```python
from build123d import *

# Parameters (mm, degrees)
SKETCH1_W           = 46
SKETCH1_H           = 42
BOSS_EXTRUDE1_DEPTH = 3
SKETCH2_W           = 13
SKETCH2_H           = 3
CUT_EXTRUDE1_DEPTH  = 32.288975694
SKETCH3_W           = 3
SKETCH3_H           = 10
CUT_EXTRUDE2_DEPTH  = 32.288975694


with BuildPart() as part:
    # Sketch1 → Boss-Extrude1 (new body)
    with BuildSketch(Plane.XY):
        Rectangle(SKETCH1_W, SKETCH1_H)
    extrude(amount=BOSS_EXTRUDE1_DEPTH)

    # Sketch2 → Cut-Extrude1 (cut, through all)
    with BuildSketch(Plane.XY.offset(3)):
        with Locations((-16.5, -19.5)):
            Rectangle(SKETCH2_W, SKETCH2_H)
        with Locations((16.5, -19.5)):
            Rectangle(SKETCH2_W, SKETCH2_H)
    extrude(amount=-CUT_EXTRUDE1_DEPTH, mode=Mode.SUBTRACT)

    # Sketch3 → Cut-Extrude2 (cut, through all)
    with BuildSketch(Plane(origin=(0, 0, 0), x_dir=(-1, 0, 0), z_dir=(0, 0, -1))):
        with Locations((-21.5, 0.5)):
            Rectangle(SKETCH3_W, SKETCH3_H)
        with Locations((21.5, 0.5)):
            Rectangle(SKETCH3_W, SKETCH3_H)
    extrude(amount=-CUT_EXTRUDE2_DEPTH, mode=Mode.SUBTRACT)


solid = part.part
```
Read the model definition and answer for the solid it produces. Units are mm, in the model's axes. A direction names the side the tool comes from. Coordinates: 2 decimals unless noted, no trailing zeros. Loops run counter-clockwise (first coordinate to the right, second up) from the corner with the lowest first, then second, coordinate; pieces in that order, holes last. Notation, with made-up numbers: (66.25, 5) - (117.25, 5) arc R7 ccw to (117.25, 14) - close; hole circle Ø5 at (63, -33.75). An arc over 180 degrees is marked (long way). Answer in a Markdown table with one row per item.
1. Which of the six approach directions +Z, -Z, +X, -X, +Y, -Y give full straight-line access (tool end or side, diameter ignored) to faces 5 (the face through (-21, -4.5, 1)), 6 (the face through (-10, -20, 2)), 7 (the face through (22, -4.5, 1))?
Conclusion:
| item | result |
|---|---|
| face 5 | +Z, -Z, -X |
| face 6 | +Z, -Z, -X, -Y |
| face 7 | +Z, -Z, +X |
2. Find section A-A, the plane z = 1. Write down the section's boundary in (x, y).
Conclusion:
| item | result |
|---|---|
| outline | (-23, -18) - (-10, -18) - (-10, -21) - (10, -21) - (10, -18) - (23, -18) - (23, -4.5) - (20, -4.5) - (20, 5.5) - (23, 5.5) - (23, 21) - (-23, 21) - (-23, 5.5) - (-20, 5.5) - (-20, -4.5) - (-23, -4.5) - close |
3. Determine the mould class of faces 1 (the face through (0, 21, 1)), 2 (the face through (10, -20, 2)), 3 (the face through (-21, 5.5, 1)), 4 (the face through (16, -18, 2)) for opening direction Y: +Y half, -Y half, draft (parallel to the pull), parting line (faces both ways), or undercut.
Conclusion:
| item | result |
|---|---|
| face 1 | +Y half |
| face 2 | draft |
| face 3 | undercut |
| face 4 | -Y half |
4. Given pin 1 (1.5 mm diameter, centred on x = 18, z = 1, fed in from -Y); pin 2 (0.9 mm diameter, centred on y = -19, z = 1, fed in from +X), each flat-ended and moving along its own axis, determine where each tip first touches the part or whether it passes through.
Conclusion:
| item | result |
|---|---|
| pin 1 | stops at y = -18 |
| pin 2 | stops at x = 10 |
5. Straight lines are drawn through the part: line 1 (Y direction, x = -10.5, z = 2.15); line 2 (X direction, y = 1, z = 1.5). For each, find the intervals that lie inside material, in ascending order.
Conclusion:
| item | result |
|---|---|
| line 1 | y = -18 to 21 |
| line 2 | x = -20 to 20 |
6. Find section B-B, the plane x = -14.5. Write down the section's boundary in (y, z), then the cut area to 3 significant figures.
Conclusion:
| item | result |
|---|---|
| outline | (-18, 0) - (21, 0) - (21, 3) - (-18, 3) - close |
| area | 117 mm² |
